```python
from build123d import *

# Parameters (mm, degrees)
SKETCH1_R           = 4.4
BOSS_EXTRUDE1_DEPTH = 10
SKETCH2_W           = 5.25
SKETCH2_H           = 5.25
BOSS_EXTRUDE2_DEPTH = 10
SKETCH3_R           = 7.5
BOSS_EXTRUDE3_DEPTH = 2


with BuildPart() as part:
    # Sketch1 → Boss-Extrude1 (new body)
    with BuildSketch(Plane.XY):
        Circle(SKETCH1_R)
    extrude(amount=BOSS_EXTRUDE1_DEPTH)

    # Sketch2 → Boss-Extrude2 (add)
    with BuildSketch(Plane.XY.offset(10)):
        Rectangle(SKETCH2_W, SKETCH2_H)
    extrude(amount=BOSS_EXTRUDE2_DEPTH)

    # Sketch3 → Boss-Extrude3 (add)
    with BuildSketch(Plane(origin=(0, 0, 0), x_dir=(-1, 0, 0), z_dir=(0, 0, -1))):
        Circle(SKETCH3_R)
    extrude(amount=BOSS_EXTRUDE3_DEPTH)


solid = part.part
```
Verification items for the finished model (mm, model axes). A direction names the side the tool comes from. Give positions to 0.01 mm unless a question says otherwise; leave off trailing zeros. Write each loop counter-clockwise with the first axis right and the second up, starting at its lowest first coordinate (ties: lowest second). Pieces come first, ordered by that corner, then holes. Notation, with made-up numbers: (30.25, -35) - (75.25, -35) arc R26 ccw to (75.25, -16) - close; hole circle Ø7 at (-3, 27.25). An arc over 180 degrees is marked (long way). Put each result on its own line as item: value.
Q1. Section check D-D on y = -3.25. Record the cut outline in (x, z).
Result:
outline: (-6.76, -2) - (6.76, -2) - (6.76, 0) - (2.97, 0) - (2.97, 10) - (-2.97, 10) - (-2.97, 0) - (-6.76, 0) - close
Q2. Section check A-A on y = 0. Record the cut outline in (x, z) (3 decimals).
Result:
outline: (-7.5, -2) - (7.5, -2) - (7.5, 0) - (4.4, 0) - (4.4, 10) - (2.625, 10) - (2.625, 20) - (-2.625, 20) - (-2.625, 10) - (-4.4, 10) - (-4.4, 0) - (-7.5, 0) - close
Q3. Section check C-C on z = 18.25. Record the cut outline in (x, y) (3 decimals), and give its area (3 significant figures).
Result:
outline: (-2.625, -2.625) - (2.625, -2.625) - (2.625, 2.625) - (-2.625, 2.625) - close
area: 27.6 mm2
Q4. Depth check by flat-ended pin: P1, Ø6, axis at y = 6, z = 9, coming from the +X side; P2, Ø1.5, axis at x = 1.5, z = 16.5, coming from the +Y side (3 decimals); P3, Ø2.5, axis at y = -1, z = 14.5, coming from the +X side (3 decimals). Enter the tip coordinate at first touch or a pass-through.
Result:
P1: x = 3.22
P2: y = 2.625
P3: x = 2.625
Q5. Scan lines: probe 1 along Z at (x, y) = (0.5, 6.75); probe 2 along Z at (x, y) = (-0.75, 3); probe 3 along X at (y, z) = (0.5, 18.5) (3 decimals). Record each from-to range of solid material in increasing order. Write a range as from..to.
Result:
probe 1: -2..0
probe 2: -2..10
probe 3: -2.625..2.625
Q6. Set-up check for faces 1 (the face through (4.197, 1.322, 4.93)), 2 (the face through (2.625, 0, 15)), 3 (the face through (0, 2.625, 15)), 4 (the face through (0, -2.625, 15)): record each of +Z, -Z, +X, -X, +Y, -Y from which the full face is reachable in a straight line by a thin tool's end or side.
Result:
face 1: +Z
face 2: +Z, +X, +Y, -Y
face 3: +Z, +X, -X, +Y
face 4: +Z, +X, -X, -Y
